from build123d import *

# Parameters (mm, degrees)
SKETCH1_R           = 8.5
BOSS_EXTRUDE1_DEPTH = 7
BOSS_EXTRUDE2_DEPTH = 0.6
SKETCH3_R           = 5.8
CUT_EXTRUDE1_DEPTH  = 4.15


with BuildPart() as part:
    # Sketch1 → Boss-Extrude1 (new body)
    with BuildSketch(Plane.XY):
        Circle(SKETCH1_R)
    extrude(amount=BOSS_EXTRUDE1_DEPTH)

    # Sketch2 → Boss-Extrude2 (add)
    with BuildSketch(Plane.XY.offset(7)):
        with BuildLine():
            Line((-3.496777173, 3.33685478), (-4.915046404, 4.853281062))
            Line((-4.915046404, 4.853281062), (-1.072898968, 4.853281062))
            Line((-1.072898968, 4.853281062), (-1.072898968, 1.123313114))
            Line((-1.072898968, 1.123313114), (-2.641408583, 2.511534267))
            add(Edge.make_bspline(
                [(-2.641408583, 2.511534267), (-2.720753384, 2.418855801), (-2.878322384, 2.234807782), (-3.080326614, 1.933878452), (-3.253390687, 1.61912069), (-3.395661366, 1.287378065), (-3.502208895, 0.938351436), (-3.581164136, 0.573998239), (-3.627606924, 0.193691534), (-3.633833749, -0.065128908), (-3.637001532, -0.196799066)],
                knots=[0, 0, 0, 0, 0.990413106, 1.966838421, 2.937869788, 3.905121185, 4.893378033, 5.897730606, 6.93050896, 8, 8, 8, 8], degree=3))
            add(Edge.make_bspline(
                [(-3.637001532, -0.196799066), (-3.633314081, -0.328490722), (-3.626080362, -0.586831876), (-3.575666424, -0.966879106), (-3.48901189, -1.329477593), (-3.370773292, -1.677822622), (-3.215507272, -2.009168524), (-3.026563561, -2.324364608), (-2.80395201, -2.623800683), (-2.549784804, -2.902253094), (-2.273703911, -3.157129382), (-1.982206578, -3.380716481), (-1.679065211, -3.570884015), (-1.361911881, -3.723224656), (-1.034237343, -3.844640529), (-0.694609323, -3.930992109), (-0.342601775, -3.981888324), (-0.104181125, -3.989174312), (0.016844622, -3.992872784)],
                knots=[0, 0, 0, 0, 1.079250243, 2.117178572, 3.135310327, 4.130457806, 5.126943688, 6.12839153, 7.13757049, 8.179760785, 9.213873081, 10.213240201, 11.186661469, 12.141254978, 13.091823965, 14.04618213, 15.008213981, 16, 16, 16, 16], degree=3))
            add(Edge.make_bspline(
                [(0.016844622, -3.992872784), (0.145225127, -3.989328055), (0.399045702, -3.982319786), (0.771483518, -3.92919274), (1.130051724, -3.842959504), (1.473171339, -3.720575099), (1.801926634, -3.562161434), (2.117866526, -3.372942158), (2.41516878, -3.142633465), (2.697195125, -2.885792453), (2.953892432, -2.602154952), (3.182127427, -2.302868546), (3.370336038, -1.984922834), (3.528939332, -1.656080542), (3.648009639, -1.310669225), (3.73821301, -0.953238154), (3.787712727, -0.57946122), (3.795125716, -0.325806083), (3.798895904, -0.196799066)],
                knots=[0, 0, 0, 0, 1.033612209, 2.043550498, 3.023051526, 3.999358907, 4.971079349, 5.957874823, 6.959200849, 7.994476354, 9.02612831, 10.03602365, 11.020045963, 11.99661988, 12.971133653, 13.957137591, 14.961016167, 16, 16, 16, 16], degree=3))
            add(Edge.make_bspline(
                [(3.798895904, -0.196799066), (3.795452622, -0.071738589), (3.788588973, 0.177550022), (3.732512198, 0.547316376), (3.642339714, 0.909630301), (3.515407262, 1.263936549), (3.351110497, 1.609595982), (3.154582121, 1.949790991), (2.919499892, 2.281514078), (2.739012005, 2.489632171), (2.647052955, 2.595668883)],
                knots=[0, 0, 0, 0, 0.970334418, 1.934210747, 2.895854909, 3.864734812, 4.850109812, 5.862644845, 6.911011974, 8, 8, 8, 8], degree=3))
            Line((2.647052955, 2.595668883), (3.524456802, 3.412976575))
            add(Edge.make_bspline(
                [(3.524456802, 3.412976575), (3.658278985, 3.275504412), (3.91937115, 3.007290997), (4.264397959, 2.578686277), (4.553163347, 2.138040406), (4.795240196, 1.68988536), (4.980930526, 1.228890741), (5.110227561, 0.756857332), (5.195045563, 0.27566711), (5.204437058, -0.049543732), (5.209152314, -0.212824707)],
                knots=[0, 0, 0, 0, 1.119978514, 2.185120635, 3.207184244, 4.192840501, 5.155195957, 6.102228941, 7.047172264, 8, 8, 8, 8], degree=3))
            add(Edge.make_bspline(
                [(5.209152314, -0.212824707), (5.204540212, -0.382014013), (5.195439592, -0.715859062), (5.12297081, -1.207015128), (5.007595574, -1.680619371), (4.842005, -2.136576039), (4.627397829, -2.574094346), (4.371358267, -2.997310094), (4.06311267, -3.39955484), (3.713795898, -3.780248165), (3.331337364, -4.130160805), (2.922899491, -4.437565389), (2.490856262, -4.694704345), (2.038857832, -4.9089885), (1.563247201, -5.073941917), (1.066251184, -5.188891521), (0.548487363, -5.261364491), (0.196039665, -5.270353687), (0.016844622, -5.274924066)],
                knots=[0, 0, 0, 0, 1.006511856, 1.986053414, 2.947928005, 3.903304009, 4.866581259, 5.843887477, 6.842136409, 7.877167342, 8.915131082, 9.922897295, 10.913810849, 11.902179308, 12.895003365, 13.90323956, 14.933943735, 16, 16, 16, 16], degree=3))
            add(Edge.make_bspline(
                [(0.016844622, -5.274924066), (-0.154981037, -5.270101549), (-0.493322306, -5.26060555), (-0.991507142, -5.1914642), (-1.470001358, -5.07522348), (-1.929693111, -4.911786456), (-2.370270316, -4.702826529), (-2.791145936, -4.446149677), (-3.192948817, -4.14431338), (-3.57070976, -3.800322782), (-3.913756475, -3.422137917), (-4.219341638, -3.023295532), (-4.474952699, -2.601787942), (-4.684175633, -2.161406889), (-4.847542361, -1.701662708), (-4.963802172, -1.22318273), (-5.032938356, -0.724994042), (-5.042435065, -0.386653302), (-5.047257942, -0.214827912)],
                knots=[0, 0, 0, 0, 1.035645246, 2.039285224, 3.025359342, 3.999339005, 4.975246586, 5.959692554, 6.966033149, 8.00039464, 9.034756131, 10.040307446, 11.024753414, 12.000660995, 12.974640658, 13.960714776, 14.964354754, 16, 16, 16, 16], degree=3))
            add(Edge.make_bspline(
                [(-5.047257942, -0.214827912), (-5.042718501, -0.042971038), (-5.033757492, 0.296280149), (-4.960307444, 0.794688321), (-4.838251028, 1.272224933), (-4.665501402, 1.727921947), (-4.449759875, 2.165386428), (-4.180027486, 2.580020601), (-3.863065273, 2.974774534), (-3.620105292, 3.214943433), (-3.496777173, 3.33685478)],
                knots=[0, 0, 0, 0, 1.032765718, 2.038713884, 3.021079012, 3.990324489, 4.963319928, 5.947610502, 6.958193293, 8, 8, 8, 8], degree=3))
        make_face()
    extrude(amount=BOSS_EXTRUDE2_DEPTH)

    # Sketch3 → Cut-Extrude1 (cut)
    with BuildSketch(Plane(origin=(0, 0, 0), x_dir=(-1, 0, 0), z_dir=(0, 0, -1))):
        Circle(SKETCH3_R)
    extrude(amount=-CUT_EXTRUDE1_DEPTH, mode=Mode.SUBTRACT)


solid = part.part
Build history of the part. All positions in model axes, mm. A direction names the side the tool comes from. Round coordinates to 2 decimals unless told otherwise and drop trailing zeros. Write each loop counter-clockwise with the first axis right and the second up, starting at its lowest first coordinate (ties: lowest second). Pieces come first, ordered by that corner, then holes. Notation, with made-up numbers: (84, 70.25) - (116, 70.25) arc R22 cw to (116, 98.25) - close; hole circle Ø7 at (-17.5, -17.5). An arc over 180 degrees is marked (long way). Use CSV: the item, a comma, the result in double quotes.
(1) Wall check: line 1 (Y direction, x = 0, z = 3.25); line 2 (Z direction, x = 5.75, y = 4.5); line 3 (Z direction, x = -4.25, y = 2). Give the ranges that are in metal, low to high.
Response:
line 1,"-8.5 to -5.8, 5.8 to 8.5"
line 2,"0 to 7"
line 3,"4.15 to 7.6"
(2) Band-saw the part on C-C (y = -7.5). Write the cut outline in (x, z).
Response:
outline,"(-4, 0) - (4, 0) - (4, 7) - (-4, 7) - close"
(3) 3-axis set-ups, long thin cutter, end or side, ignore diameter. For faces 1 (the flat face through (-4.196, 4.084, 7.296)), 2 (the flat face through (2, -6, 0)), 3 (the flat face through (3.08, 3, 7.3)), 4 (the flat face through (0, 0, 7)), 5 (the cylindrical face through (5.794, 0.255, 2.046)): which of +Z, -Z, +X, -X, +Y, -Y reach the whole face in a straight line?
Response:
face 1,"+Z, -X"
face 2,"-Z, +X, -X, +Y, -Y"
face 3,"+Z, +Y"
face 4,"+Z"
face 5,"-Z"
(4) Pin check, flat tips, straight feed: P1, Ø0.7, axis at y = 3, z = 7, coming from the +X side; P2, Ø5, axis at x = -3, y = -1, coming from the -Z side; P3, Ø1, axis at x = 0, y = -6.5, coming from the +Z side. Stop position of each tip, or through.
Response:
P1,"x = 8.08"
P2,"z = 4.15"
P3,"z = 7"
(5) Band-saw the part on A-A (z = 3). Write the cut outline in (x, y), plus the area to 3 significant figures.
Response:
outline,"circle Ø17 at (0, 0); hole circle Ø11.6 at (0, 0)"
area,"121 mm²"
(6) Mould opens along X. For faces 6 (the flat face through (-1.85, 1.81, 7.3)), 7 (the flat face through (-1.4, 2.1, 7.6)), 8 (the cylindrical face through (4.57, 7.167, 3.451)) say: pulls with the +X half, pulls with the -X half, needs draft (parallel to the pull), parting line crosses it, or undercut.
Response:
face 6,"undercut"
face 7,"needs draft"
face 8,"parting line crosses it"
(7) Band-saw the part on B-B (x = -5.25). Write the cut outline in (y, z).
Response:
outline,"(-6.68, 0) - (-2.47, 0) - (-2.47, 4.15) - (2.47, 4.15) - (2.47, 0) - (6.68, 0) - (6.68, 7) - (-6.68, 7) - close"
(8) Band-saw the part on D-D (z = 4.5). Write the cut outline in (x, y).
Response:
outline,"circle Ø17 at (0, 0)"
